```python
from build123d import *

# Parameters (mm, degrees)
SKETCH_R     = 1.5
PAD_DEPTH    = 6
SKETCH001_W  = 4.2
SKETCH001_H  = 1.6
POCKET_DEPTH = 5
FILLET_R     = 2
FILLET001_R  = 0.7
PAD001_DEPTH = 2


with BuildPart() as part:
    # Sketch → Pad (new body)
    with BuildSketch(Plane.XY):
        with BuildLine():
            ThreePointArc((2.44949, -0.5), (-1.581139, 1.936492), (0, -2.5))
            Line((0, -2.5), (11.5, -2.5))
            Line((11.5, -2.5), (11.5, -0.5))
            Line((11.5, -0.5), (2.44949, -0.5))
        make_face()
        Circle(SKETCH_R, mode=Mode.SUBTRACT)
    extrude(amount=PAD_DEPTH)

    # Sketch001 (on Face2 of Pad) → Pocket (cut)
    with BuildSketch(Plane.XZ.offset(2.5)):
        with Locations((7.8, 3.064189)):
            Rectangle(SKETCH001_W, SKETCH001_H)
    extrude(amount=-POCKET_DEPTH, mode=Mode.SUBTRACT)

    # Fillet
    fillet_edges = [part.edges().sort_by_distance(p)[0] for p in [
        (11.5, -1.5, 6),
        (11.5, -1.5, 0),
    ]]
    fillet(fillet_edges, radius=FILLET_R)

    # Fillet001
    fillet001_edges = [part.edges().sort_by_distance(p)[0] for p in [
        (5.7, -1.5, 3.864189),
        (5.7, -1.5, 2.264189),
        (9.9, -1.5, 3.864189),
        (9.9, -1.5, 2.264189),
    ]]
    fillet(fillet001_edges, radius=FILLET001_R)

    # Sketch002 (on Face16 of Fillet001) → Pad001 (join)
    with BuildSketch(Plane.XZ.offset(2.5)):
        with BuildLine():
            Line((6.359142, 3.664189), (9.14113, 3.664189))
            Line((9.14113, 3.664189), (9.14113, 2.414189))
            Line((9.14113, 2.414189), (11.049985, 0.577696))
            ThreePointArc((11.049985, 0.577696), (11.316274, 0.938609), (11.5, 1.347771))
            Line((11.5, 1.347771), (11.5, 0))
            Line((11.5, 0), (10.152229, 0))
            ThreePointArc((10.152229, 0), (10.603745, 0.209148), (10.993504, 0.518497))
            Line((10.993504, 0.518497), (9.023117, 2.414189))
            Line((9.023117, 2.414189), (6.359142, 2.414189))
            Line((6.359142, 2.414189), (6.359142, 3.664189))
        make_face()
    extrude(amount=-PAD001_DEPTH)


solid = part.part
```
Check sheet for the modelled part. Datum: model origin and axes. Units: mm. A direction names the side the tool comes from. Give positions to 0.01 mm unless a question says otherwise; leave off trailing zeros. Loops run counter-clockwise (first coordinate to the right, second up) from the corner with the lowest first, then second, coordinate; pieces in that order, holes last. Notation, with made-up numbers: M 27.5,-39 L 38.5,-39 A5 ccw 38.5,-35 Z; hole C 17.5,45.25 d7. An arc over 180 degrees is marked long. Answer in a Markdown table with one row per item.
1) Cross-section at B-B (y = -0.9). Count the separate pieces of the cut face and the enclosed holes in it, plus the area to 3 significant figures.
Solutions:
| item | result |
|---|---|
| separate pieces | 2 |
| enclosed holes | 1 |
| area | 64.7 mm^2 |
2) Depth check by flat-ended pin: pin 1 (0.6 mm diameter, centred on y = -1, z = 3, fed in from -X). Enter the tip coordinate at first touch or a pass-through.
Solutions:
| item | result |
|---|---|
| pin 1 | stops at x = -2.4 |
3) Thickness scan on line 1 (Y direction, x = 0, z = 1.5); line 2 (Y direction, x = 4.5, z = 4.25); line 3 (X direction, y = -0.8, z = 2.45). Record the ranges inside material, lowest first.
Solutions:
| item | result |
|---|---|
| line 1 | y = -2.5 to -1.5, 1.5 to 2.5 |
| line 2 | y = -2.5 to -0.5 |
| line 3 | x = -2.37 to -1.27, 1.27 to 5.93, 6.36 to 9.14, 9.67 to 11.5 |
4) Cross-section at D-D (z = 1.2). Enter the section's corners in (x, y), plus the area to 3 significant figures.
Solutions:
| item | result |
|---|---|
| outline | M 0,-2.5 L 11.33,-2.5 L 11.33,-0.5 L 2.45,-0.5 A2.5 ccw long Z; M 11.45,-2.5 L 11.5,-2.5 L 11.5,-0.5 L 11.45,-0.5 Z; hole C 0,0 d3 |
| area | 31.7 mm^2 |
5) Cross-section at C-C (y = 0). Enter the section's corners in (x, z), plus the area to 3 significant figures.
Solutions:
| item | result |
|---|---|
| outline | M -2.5,0 L -1.5,0 L -1.5,6 L -2.5,6 Z; M 1.5,0 L 2.5,0 L 2.5,6 L 1.5,6 Z |
| area | 12.0 mm^2 |
6) Tool access check on faces 4 (the face through (6, -2.5, 2)), 5 (the face through (8, -2, 3.864)). Record the directions out of +Z, -Z, +X, -X, +Y, -Y that give a thin tool (end or side, any length) a straight path to the whole face; none if there is none.
Solutions:
| item | result |
|---|---|
| face 4 | +Z, -Z, +X, -X, -Y |
| face 5 | +Y, -Y |
7) Cross-section at A-A (z = 3.35). Enter the section's corners in (x, y).
Solutions:
| item | result |
|---|---|
| outline | M 0,-2.5 L 5.73,-2.5 L 5.73,-0.5 L 2.45,-0.5 A2.5 ccw long Z; M 6.36,-2.5 L 9.14,-2.5 L 9.14,-0.5 L 6.36,-0.5 Z; M 9.87,-2.5 L 11.5,-2.5 L 11.5,-0.5 L 9.87,-0.5 Z; hole C 0,0 d3 |
8) Mould release check, pull along X, two halves, no side actions. Record for faces 1 (the face through (-1.5, 0.07, 2.96)), 2 (the face through (11.5, -2, 3)), 3 (the face through (3, -1, 6)): released by +X, released by -X, zero draft, split by the parting line, or undercut.
Solutions:
| item | result |
|---|---|
| face 1 | undercut |
| face 2 | released by +X |
| face 3 | zero draft |
